from build123d import *

# Parameters (mm, degrees)
BOSS_EXTRUDE1_DEPTH  = 10.5
SKETCH2_R            = 1.25
CUT_EXTRUDE1_DEPTH   = 46.038983115
BOSS_EXTRUDE19_DEPTH = 1.2
LPATTERN1_START      = -6.7
LPATTERN1_DEPTH      = 2.4
LPATTERN1_START_2    = 4.3
LPATTERN1_2_DEPTH    = 2.4
SKETCH5_R            = 3
CUT_EXTRUDE2_DEPTH   = 2.5
FILLET1_R            = 1
BOSS_EXTRUDE20_DEPTH = 5
FILLET2_R            = 1
BOSS_EXTRUDE21_DEPTH = 2.5


# Read off the part's stored shape, not the designer's step: LPattern1
with BuildPart() as part:
    # Sketch1 → Boss-Extrude1 (new, symmetric)
    with BuildSketch(Plane.XY):
        Polygon((-43.5, 2.6), (-16.5, 2.6), (-14, 0), (14, 0), (16.5, 2.6), (43.5, 2.6), (43.5, 5.1), (16, 5.1), (13.5, 2.6), (-13.5, 2.6), (-16, 5.1), (-43.5, 5.1), align=None)
    extrude(amount=BOSS_EXTRUDE1_DEPTH, both=True)

    # Sketch2 → Cut-Extrude1 (cut, through all)
    with BuildSketch(Plane(origin=(0, 5.1, 0), x_dir=(1, 0, 0), z_dir=(0, 1, 0))):
        with Locations(Location((27, 0, 0), (0, 0, 180))):
            Circle(SKETCH2_R)
        with Locations(Location((41.7, 0, 0), (0, 0, 180))):
            Circle(SKETCH2_R)
    cut_extrude1 = extrude(amount=-CUT_EXTRUDE1_DEPTH, mode=Mode.SUBTRACT)

    # Mirror1: Cut-Extrude1 across plane
    add(cut_extrude1.mirror(Plane(origin=(0, 0, 0), x_dir=(0, 0, 1), z_dir=(1, 0, 0))), mode=Mode.SUBTRACT)

    # Sketch4 → Boss-Extrude19 (add, symmetric)
    with BuildSketch(Plane.XY):
        Polygon((-43.5, 7.6), (-14.587766262, 7.6), (-12.087766262, 5.1), (12.087766262, 5.1), (14.587766262, 7.6), (43.5, 7.6), (43.5, 5.1), (16, 5.1), (13.5, 2.6), (-13.5, 2.6), (-16, 5.1), (-43.5, 5.1), align=None)
    boss_extrude19 = extrude(amount=BOSS_EXTRUDE19_DEPTH, both=True)

    # Mirror2: Boss-Extrude19 across plane
    add(boss_extrude19.mirror(Plane.XY))

    # LPattern1 outline → LPattern1 (add)
    with BuildSketch(Plane.XY.offset(LPATTERN1_START)):
        Polygon((14.587766262, 7.6), (12.087766262, 5.1), (-12.087766262, 5.1), (-14.587766262, 7.6), (-43.5, 7.6), (-43.5, 5.1), (-16, 5.1), (-13.5, 2.6), (13.5, 2.6), (16, 5.1), (43.5, 5.1), (43.5, 7.6), align=None)
    extrude(amount=LPATTERN1_DEPTH)

    # LPattern1 2 outline → LPattern1 2 (add)
    with BuildSketch(Plane.XY.offset(LPATTERN1_START_2)):
        Polygon((14.587766262, 7.6), (12.087766262, 5.1), (-12.087766262, 5.1), (-14.587766262, 7.6), (-43.5, 7.6), (-43.5, 5.1), (-16, 5.1), (-13.5, 2.6), (13.5, 2.6), (16, 5.1), (43.5, 5.1), (43.5, 7.6), align=None)
    extrude(amount=LPATTERN1_2_DEPTH)

    # Sketch5 → Cut-Extrude2 (cut)
    with BuildSketch(Plane(origin=(0, 7.6, 0), x_dir=(1, 0, 0), z_dir=(0, 1, 0))):
        with Locations((-41.7, 0)):
            Circle(SKETCH5_R)
        with Locations((-27, 0)):
            Circle(SKETCH5_R)
        with Locations((42.888677457, 0)):
            Circle(SKETCH5_R)
        with Locations((28.188677457, 0)):
            Circle(SKETCH5_R)
    extrude(amount=-CUT_EXTRUDE2_DEPTH, mode=Mode.SUBTRACT)

    # Fillet1
    fillet1_edges = [part.edges().sort_by_distance(p)[0] for p in [
        (-29.749545417, 6.35, -1.2),
        (-24.250454583, 6.35, -1.2),
        (40.13913204, 6.35, -1.2),
        (25.43913204, 6.35, -1.2),
        (30.938222874, 6.35, -1.2),
        (-38.950454583, 6.35, -1.2),
        (-38.950454583, 6.35, 1.2),
        (30.938222874, 6.35, 1.2),
        (25.43913204, 6.35, 1.2),
        (40.13913204, 6.35, 1.2),
        (-24.250454583, 6.35, 1.2),
        (-29.749545417, 6.35, 1.2),
    ]]
    fillet(fillet1_edges, radius=FILLET1_R)

    # Sketch6 → Boss-Extrude20 (add)
    with BuildSketch(Plane(origin=(0, 7.6, 0), x_dir=(1, 0, 0), z_dir=(0, 1, 0))):
        with BuildLine():
            Line((43.5, -4.3), (43.5, -6.7))
            Line((43.5, -6.7), (44.75, -6.7))
            ThreePointArc((44.75, -6.7), (45.95, -5.5), (44.75, -4.3))
            Line((44.75, -4.3), (43.5, -4.3))
        make_face()
        with BuildLine():
            Line((43.5, 6.7), (43.5, 4.3))
            Line((43.5, 4.3), (44.75, 4.3))
            ThreePointArc((44.75, 4.3), (45.95, 5.5), (44.75, 6.7))
            Line((44.75, 6.7), (43.5, 6.7))
        make_face()
        with BuildLine():
            Line((-43.5, 6.7), (-44.75, 6.7))
            ThreePointArc((-44.75, 6.7), (-45.95, 5.5), (-44.75, 4.3))
            Line((-44.75, 4.3), (-43.5, 4.3))
            Line((-43.5, 4.3), (-43.5, 6.7))
        make_face()
        with BuildLine():
            Line((-43.5, -4.3), (-44.75, -4.3))
            ThreePointArc((-44.75, -4.3), (-45.95, -5.5), (-44.75, -6.7))
            Line((-44.75, -6.7), (-43.5, -6.7))
            Line((-43.5, -6.7), (-43.5, -4.3))
        make_face()
    extrude(amount=-BOSS_EXTRUDE20_DEPTH)

    # Fillet2
    fillet2_edges = [part.edges().sort_by_distance(p)[0] for p in [
        (43.5, 3.85, 10.5),
        (-43.5, 3.85, 10.5),
        (43.5, 3.85, -10.5),
        (-43.5, 3.85, -10.5),
    ]]
    fillet(fillet2_edges, radius=FILLET2_R)

    # Sketch7 → Boss-Extrude21 (add)
    with BuildSketch(Plane(origin=(0, 5.1, 0), x_dir=(1, 0, 0), z_dir=(0, 1, 0))):
        with BuildLine():
            Line((43.5, -2.079062289), (43.5, 2.079062289))
            ThreePointArc((43.5, 2.079062289), (44.45, 0), (43.5, -2.079062289))
        make_face()
        with BuildLine():
            Line((-43.5, -2.079062289), (-43.5, 2.079062289))
            ThreePointArc((-43.5, 2.079062289), (-44.45, 0), (-43.5, -2.079062289))
        make_face()
    extrude(amount=-BOSS_EXTRUDE21_DEPTH)


solid = part.part
Work out the finished part from the listing and answer in its coordinate system (mm). A direction names the side the tool comes from. Give positions to 0.01 mm unless a question says otherwise; leave off trailing zeros. Loops run counter-clockwise (first coordinate to the right, second up) from the corner with the lowest first, then second, coordinate; pieces in that order, holes last. Notation, with made-up numbers: (-23, 79.25) -> (10, 79.25) arc R24 ccw to (10, 94.25) -> close; hole circle Ø4 at (77, 53.5). An arc over 180 degrees is marked (long way). Use a Markdown table: item, result. Add a question column.
1. Section C-C on x = 5 is taken. Determine the outline of the cut face in (y, z), and give its area (3 significant figures).
2. Flat-ended cylindrical pins translate along their axes: pin 1 Ø2.5 at (x, y) = (7, 6) entering from +Z; pin 2 Ø2.5 at (x, z) = (-5, 6) entering from +Y; pin 3 Ø2 at (y, z) = (4, -8.5) entering from +X. Find the tip coordinate at first contact, or state that the pin passes through.
3. Find the intervals of material crossed by probe 1 along Z at (x, y) = (34, 7); probe 2 along Z at (x, y) = (-41.7, 3.4); probe 3 along Y at (x, z) = (-34.5, 2), in increasing order.
4. Section D-D on y = 1.5 is taken. Determine the outline of the cut face in (x, z).
5. For faces 1 (the flat face through (43.5, 4, -3)), 2 (the flat face through (-34, 6, -1.2)), 3 (the flat face through (0.9, 4.6, 1.2)), 4 (the flat face through (0, 5.1, -6)), 5 (the flat face through (-43.5, 4, 3)), determine the directions among +Z, -Z, +X, -X, +Y, -Y from which every point of the face is accessible in a straight line to the end or side of a thin tool.
6. Section B-B on z = 5.5 is taken. Determine the outline of the cut face in (x, y), and give its area (3 significant figures).
7. Section A-A on x = 27 is taken. Determine the outline of the cut face in (y, z), and give its area (4 significant figures).
8. Determine the mould class of faces 6 (the flat face through (-43.5, 4, -8)), 7 (the flat face through (30, 5.1, 9)), 8 (the flat face through (0.6, 4.6, 4.3)) for opening direction X: released by +X, released by -X, zero draft, split by the parting line, or undercut.
Results below:
| question | item | result |
|---|---|---|
| 1 | outline | (0, -10.5) -> (2.6, -10.5) -> (2.6, -6.7) -> (5.1, -6.7) -> (5.1, -4.3) -> (2.6, -4.3) -> (2.6, -1.2) -> (5.1, -1.2) -> (5.1, 1.2) -> (2.6, 1.2) -> (2.6, 4.3) -> (5.1, 4.3) -> (5.1, 6.7) -> (2.6, 6.7) -> (2.6, 10.5) -> (0, 10.5) -> close |
| 1 | area | 72.6 mm^2 |
| 2 | pin 1 | stops at z = 6.7 |
| 2 | pin 2 | stops at y = 5.1 |
| 2 | pin 3 | stops at x = 43.5 |
| 3 | probe 1 | z = -6.7 to -4.3, -1.2 to 1.2, 4.3 to 6.7 |
| 3 | probe 2 | z = -10.5 to -1.25, 1.25 to 10.5 |
| 3 | probe 3 | y = 2.6 to 5.1 |
| 4 | outline | (-15.44, -10.5) -> (15.44, -10.5) -> (15.44, 10.5) -> (-15.44, 10.5) -> close |
| 5 | face 1 | +X, +Y, -Y |
| 5 | face 2 | +X, -X, +Y |
| 5 | face 3 | +Y |
| 5 | face 4 | +Z, -Z, +Y |
| 5 | face 5 | -X, +Y, -Y |
| 6 | outline | (-45.95, 2.6) -> (-16.5, 2.6) -> (-14, 0) -> (14, 0) -> (16.5, 2.6) -> (45.95, 2.6) -> (45.95, 7.6) -> (14.59, 7.6) -> (12.09, 5.1) -> (-12.09, 5.1) -> (-14.59, 7.6) -> (-45.95, 7.6) -> close |
| 6 | area | 472 mm^2 |
| 7 | outline | (2.6, -10.5) -> (5.1, -10.5) -> (5.1, -6.7) -> (7.6, -6.7) -> (7.6, -4.3) -> (5.1, -4.3) -> (5.1, -1.25) -> (2.6, -1.25) -> close; (2.6, 1.25) -> (5.1, 1.25) -> (5.1, 4.3) -> (7.6, 4.3) -> (7.6, 6.7) -> (5.1, 6.7) -> (5.1, 10.5) -> (2.6, 10.5) -> close |
| 7 | area | 58.25 mm^2 |
| 8 | face 6 | released by -X |
| 8 | face 7 | zero draft |
| 8 | face 8 | undercut |
